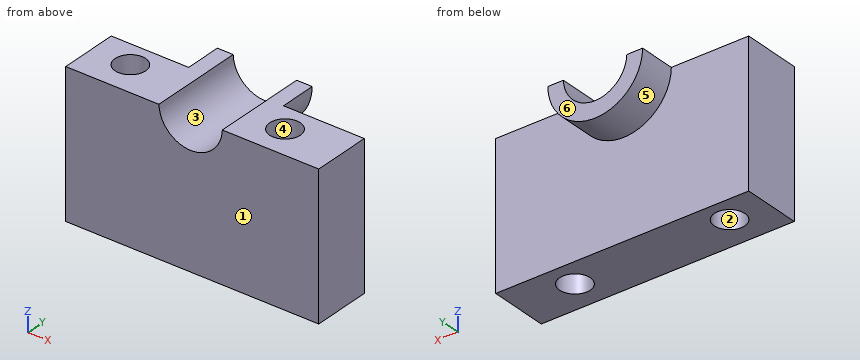
```python
from build123d import *

# Parameters (mm, degrees)
F1_DEPTH = 25.4
F3_DEPTH = 41.402
F4_R     = 6.626183
F6_DEPTH = 212.598
F5_R     = 6.659783
F7_DEPTH = 146.05


with BuildPart() as f1:
    # F0 (on Front) → F1 (new body)
    with BuildSketch(Plane.XZ):
        with BuildLine():
            Line((-17.790243, 36.410082), (-51.342823, 36.410082))
            Line((-51.342823, 36.410082), (-51.342823, -25.717501))
            Line((-51.342823, -25.717501), (58.348302, -25.717501))
            Line((58.348302, -25.717501), (58.348302, 36.410082))
            Line((58.348302, 36.410082), (23.320885, 36.410082))
            ThreePointArc((23.320885, 36.410082), (2.765321, 16.062069), (-17.790243, 36.410082))
        make_face()
    extrude(amount=F1_DEPTH)

    # F2 (on face) → F3 (join)
    with BuildSketch(Plane.XZ.offset(25.4)):
        with BuildLine():
            Line((-10.932595, 36.410082), (-17.790243, 36.410082))
            ThreePointArc((-17.790243, 36.410082), (2.765321, 16.062069), (23.320885, 36.410082))
            Line((23.320885, 36.410082), (16.566781, 36.410082))
            ThreePointArc((16.566781, 36.410082), (2.817093, 23.073848), (-10.932595, 36.410082))
        make_face()
    extrude(amount=-F3_DEPTH)

    # F4 (on face) → F6 (cut)
    with BuildSketch(Plane.XY.offset(36.410082)):
        with Locations((-34.610964, -10.85051)):
            Circle(F4_R)
    extrude(amount=-F6_DEPTH, mode=Mode.SUBTRACT)

    # F5 (on face) → F7 (cut)
    with BuildSketch(Plane.XY.offset(36.410082)):
        with Locations((33.094294, -11.707598)):
            Circle(F5_R)
    extrude(amount=-F7_DEPTH, mode=Mode.SUBTRACT)


solid = f1.part
```
Verification items for the finished model (mm, model axes). Face numbers are marked on the shaded views. A direction names the side the tool comes from. Round coordinates to 2 decimals unless told otherwise and drop trailing zeros. Order: outer loops, then holes, each group sorted by start corner. A loop starts at its lowest first (then second) coordinate and runs counter-clockwise, first axis right, second up. Notation, with made-up numbers: (-13, 38) - (16, 38) arc R19 ccw to (16, 59) - close; hole circle Ø6 at (48.5, 41.5). An arc over 180 degrees is marked (long way). Use CSV: the item, a comma, the result in double quotes. Start each with the question number.
1) Go/stop test with flat-tipped pins: P1, Ø3, axis at x = -26, z = -2.5, coming from the +Y side; P2, Ø10.5, axis at x = 33.09, y = -11.71, coming from the -Z side. Record where each tip stops, or that it passes through.
2) Thickness scan on L1, parallel to X at y = -14.5, z = -1.5; L2, parallel to X at y = -10, z = -19; L3, parallel to Y at x = -15.5, z = 7.5. Record the ranges inside material, lowest first.
3) Mould release check, pull along Y, two halves, no side actions. Record for the marked faces 1, 2, 3 and 4: +Y half, -Y half, draft (parallel to the pull), parting line (faces both ways), or undercut.
4) Section check B-B, the plane x = 29.5. Record the cut outline in (y, z), plus the area to 3 significant figures.
5) Section check A-A, the plane z = 25. Record the cut outline in (x, y).
6) Section check C-C, the plane z = -20.5. Record the cut outline in (x, y).
7) Access from +Z, -Z, +X, -X, +Y, -Y to the whole of each face (thin tool, end or side, straight path). Record for the marked faces 5 and 6.
8) Section check D-D, the plane y = -20.5. Record the cut outline in (x, z), plus the area to 3 significant figures.
Answers:
1,P1,"stops at y = 0"
1,P2,"passes through"
2,L1,"x = -51.34 to -40.14, -29.08 to 27.05, 39.14 to 58.35"
2,L2,"x = -51.34 to -41.18, -28.04 to 26.66, 39.53 to 58.35"
2,L3,"y = -25.4 to 0"
3,face 1,"-Y half"
3,face 2,"undercut"
3,face 3,"draft"
3,face 4,"undercut"
4,outline,"(-25.4, -25.72) - (-17.31, -25.72) - (-17.31, 36.41) - (-25.4, 36.41) - close; (-6.1, -25.72) - (0, -25.72) - (0, 36.41) - (-6.1, 36.41) - close"
4,area,"881 mm²"
5,outline,"(-51.34, -25.4) - (-4.2, -25.4) - (-4.2, 16) - (-14.19, 16) - (-14.19, 0) - (-51.34, 0) - close; (9.84, -25.4) - (58.35, -25.4) - (58.35, 0) - (19.72, 0) - (19.72, 16) - (9.84, 16) - close; hole circle Ø13.25 at (-34.61, -10.85); hole circle Ø13.32 at (33.09, -11.71)"
6,outline,"(-51.34, -25.4) - (58.35, -25.4) - (58.35, 0) - (-51.34, 0) - close; hole circle Ø13.25 at (-34.61, -10.85); hole circle Ø13.32 at (33.09, -11.71)"
7,face 5,"-Z, +Y"
7,face 6,"+Z, -Z, +X, -X, +Y"
8,outline,"(-51.34, -25.72) - (58.35, -25.72) - (58.35, 36.41) - (16.57, 36.41) arc R13.76 cw to (-10.93, 36.41) - (-51.34, 36.41) - close"
8,area,"6,530 mm²"
